Check sheet for the modelled part. Datum: model origin and axes. Units: mm. A direction names the side the tool comes from. Coordinates: 2 decimals unless noted, no trailing zeros. Loops run counter-clockwise (first coordinate to the right, second up) from the corner with the lowest first, then second, coordinate; pieces in that order, holes last. Notation, with made-up numbers: (11, 89.25) - (55, 89.25) arc R28 ccw to (55, 116.25) - close; hole circle Ø1 at (58.5, 20.5). An arc over 180 degrees is marked (long way). Write each question's results on one line, items separated by ' | '. Start each with the question number.
1. Cross-section at D-D (y = -1.5). Record the cut outline in (x, z), and give its area (3 significant figures).
2. Draft check along X on faces 1 (the face through (-1.715, 0.245, -0.301)), 2 (the face through (23.699, -6.853, -2.285)), 3 (the face through (-7, 0, -18)). Enter one of: released by +X, released by -X, zero draft, split by the parting line, or undercut.
3. Thickness scan on line 1 (Y direction, x = 31.5, z = -16.7); line 2 (Y direction, x = 12, z = -1); line 3 (X direction, y = -2.5, z = -16.5). Record the ranges inside material, lowest first. Write a range as [from, to].
4. Cross-section at B-B (y = 10.25). Record the cut outline in (x, z).
5. Gauge pin test, flat ends, axial feed: P1, Ø1.5, axis at y = 7, z = -11, coming from the -X side; P2, Ø7, axis at x = -7.5, y = -10.25, coming from the +Z side; P3, Ø10, axis at y = -8, z = -4, coming from the +X side; P4, Ø4, axis at x = 31.5, y = 10.25, coming from the +Z side. Record the tip position at first contact, or that the pin passes through.
6. Tool access check on faces 4 (the face through (-8, 0, -16)), 5 (the face through (12, -7, -2)), 6 (the face through (12, 3.5, -1)), 7 (the face through (26, 0, -8)). Record the directions out of +Z, -Z, +X, -X, +Y, -Y that give a thin tool (end or side, any length) a straight path to the whole face; none if there is none.
7. Cross-section at A-A (z = -10.5). Record the cut outline in (x, y), and give its area (3 significant figures).
8. Cross-section at C-C (x = -7.5). Record the cut outline in (y, z).
Solid Edge part; units mm, degrees
sketch "Sketch1" plane through (0, 0, 0) normal (0, -1, 0) x (1, 0, 0)
  line L0 (24, -18) -> (24, -2)
  line L1 (0, -2) -> (24, -2)
  line L2 (0, -18) -> (0, -2)
  line L3 (-2, -18) -> (0, -18)
  line L4 (-2, -18) -> (-12, -18)
  line L5 (-12, -18) -> (-12, -16)
  line L6 (-12, -16) -> (-2, -16)
  line L7 (-2, -16) -> (-2, 0)
  line L8 (-2, 0) -> (26, 0)
  line L9 (26, -16) -> (26, 0)
  line L10 (26, -16) -> (36, -16)
  line L11 (36, -16) -> (36, -18)
  line L12 (24, -18) -> (36, -18)
extrude "Protrusion1" add sketch "Sketch1" along normal mid plane 35
fillet "CurvePart" radius 1 1 edges at (26, 0, 0)
fillet "CurvePart2" radius 1 1 edges at (-2, 0, 0)
fillet "CurvePart3" radius 1 1 edges at (-2, 0, -16)
fillet "CurvePart4" radius 1 1 edges at (0, 0, -18)
fillet "CurvePart5" radius 1 1 edges at (24, 0, -18)
fillet "CurvePart6" radius 1 1 edges at (26, 0, -16)
fillet "CurvePart7" radius 1 1 edges at (0, 0, -2)
fillet "CurvePart8" radius 1 1 edges at (24, 0, -2)
sketch "Sketch2" plane through (12, 0, 0) normal (0, 0, 1) x (0, -1, 0)
  line L0 (-17.5, -12) -> (-3.5, -12)
  line L1 (-3.5, -12) -> (-3.5, 12)
  line L2 (-3.5, 12) -> (-17.5, 12)
  line L3 (-17.5, 12) -> (-17.5, -12)
extrude "CutOffTopPart" cut sketch "Sketch2" against normal blind 4
sketch "Sketch3" plane through (-7.5, 0, -16) normal (0, 0, 1) x (0, -1, 0)
  circle A0 centre (-10.25, 0) radius 2.25
  circle A1 centre (10.25, 0) radius 2.25
extrude "v_2Holes_Left" cut sketch "Sketch3" against normal blind 2
sketch "Sketch4" plane through (31.5, 0, -16) normal (0, 0, 1) x (1, 0, 0)
  circle A0 centre (0, -10.25) radius 2.25
  circle A1 centre (0, 10.25) radius 2.25
extrude "v_2Holes_Right" cut sketch "Sketch4" against normal blind 2
sketch "Sketch5" plane through (12, 0, 0) normal (0, 0, 1) x (1, 0, 0)
  circle A0 centre (0, -1.5) radius 2.25
  circle A1 centre (0, -9.5) radius 2.25
extrude "v_2Holes_Middle" cut sketch "Sketch5" against normal blind 2
Established:
1) outline: (-12, -18) - (-1, -18) arc R1 ccw to (0, -17) - (0, -3) arc R1 cw to (1, -2) - (9.75, -2) - (9.75, 0) - (-1, 0) arc R1 ccw to (-2, -1) - (-2, -15) arc R1 cw to (-3, -16) - (-12, -16) - close; (14.25, -2) - (23, -2) arc R1 cw to (24, -3) - (24, -17) arc R1 ccw to (25, -18) - (36, -18) - (36, -16) - (27, -16) arc R1 cw to (26, -15) - (26, -1) arc R1 ccw to (25, 0) - (14.25, 0) - close | area: 151 mm^2
2) face 1: released by -X | face 2: undercut | face 3: zero draft
3) line 1: [-17.5, -12.5], [-8, 8], [12.5, 17.5] | line 2: [-17.5, -11.75], [-7.25, -3.75], [0.75, 3.5] | line 3: [-12, 0], [24, 36]
4) outline: (-12, -18) - (-9.75, -18) - (-9.75, -16) - (-12, -16) - close; (-5.25, -18) - (-1, -18) arc R1 ccw to (0, -17) - (0, 0) - (-1, 0) arc R1 ccw to (-2, -1) - (-2, -15) arc R1 cw to (-3, -16) - (-5.25, -16) - close; (24, -17) arc R1 ccw to (25, -18) - (29.25, -18) - (29.25, -16) - (27, -16) arc R1 cw to (26, -15) - (26, -1) arc R1 ccw to (25, 0) - (24, 0) - close; (33.75, -18) - (36, -18) - (36, -16) - (33.75, -16) - close
5) P1: x = -2 | P2: z = -16 | P3: x = 26 | P4: through
6) face 4: +Z, -X, +Y, -Y | face 5: -Z, +Y, -Y | face 6: +Z, -Z, +Y | face 7: +Z, +X, +Y, -Y
7) outline: (-2, -17.5) - (0, -17.5) - (0, 17.5) - (-2, 17.5) - close; (24, -17.5) - (26, -17.5) - (26, 17.5) - (24, 17.5) - close | area: 140 mm^2
8) outline: (-17.5, -18) - (-12.5, -18) - (-12.5, -16) - (-17.5, -16) - close; (-8, -18) - (8, -18) - (8, -16) - (-8, -16) - close; (12.5, -18) - (17.5, -18) - (17.5, -16) - (12.5, -16) - close
